from build123d import *

# Parameters (mm, degrees)
SKETCH_1_W          = 40
SKETCH_1_H          = 70
EXTRUDE_1_DEPTH     = 3
SKETCH_2_R          = 1.5
CUT_EXTRUDE_1_DEPTH = 3
CHAMFER_1_SIZE      = 0.5
CUT_EXTRUDE_2_DEPTH = 3


with BuildPart() as part:
    # 草图1 → 凸台-拉伸1 (new body)
    with BuildSketch(Plane(origin=(0, 0, 0), x_dir=(1, 0, 0), z_dir=(0, 1, 0))):
        Rectangle(SKETCH_1_W, SKETCH_1_H)
    extrude(amount=EXTRUDE_1_DEPTH)

    # 草图2 → 切除-拉伸1 (cut)
    with BuildSketch(Plane(origin=(0, 3, 0), x_dir=(1, 0, 0), z_dir=(0, 1, 0))):
        with Locations(Location((-17, 32, 0), (0, 0, 270))):
            Circle(SKETCH_2_R)
        with Locations(Location((-17, -32, 0), (0, 0, 270))):
            Circle(SKETCH_2_R)
        with Locations(Location((17, 32, 0), (0, 0, 270))):
            Circle(SKETCH_2_R)
        with Locations(Location((17, -32, 0), (0, 0, 270))):
            Circle(SKETCH_2_R)
    extrude(amount=-CUT_EXTRUDE_1_DEPTH, mode=Mode.SUBTRACT)

    # 倒角1
    chamfer_1_edges = [part.edges().sort_by_distance(p)[0] for p in [
        (-17, 0, 30.5),
        (17, 0, -33.5),
        (17, 0, 30.5),
        (-17, 0, -33.5),
    ]]
    chamfer(chamfer_1_edges, length=CHAMFER_1_SIZE)

    # 草图3 → 切除-拉伸2 (cut)
    with BuildSketch(Plane(origin=(0, 3, 0), x_dir=(1, 0, 0), z_dir=(0, 1, 0))):
        Polygon((-17, 28), (-17, 5), (-3, 28), align=None)
        Polygon((-2.622834476, 20.926536493), (-6.262463104, 14.947146604), (-2.622834476, 12.731720482), align=None)
        Polygon((-8.320477478, 12.687787001), (-2.483236099, 9.134683552), (-5, 5), (-13, 5), align=None)
        Polygon((-2.032840116, 6.708397111), (-3.07273401, 5), (-2.032840116, 5), align=None)
        Polygon((3.07273401, 5), (2.032840116, 5), (2.032840116, 6.708397111), align=None)
        Polygon((5, 5), (13, 5), (8.320477478, 12.687787001), (2.483236099, 9.134683552), align=None)
        Polygon((6.262463104, 14.947146604), (2.622834476, 12.731720482), (2.622834476, 20.926536493), align=None)
        Polygon((17, 5), (3, 28), (17, 28), align=None)
        Polygon((2.032840116, -6.708397111), (3.07273401, -5), (2.032840116, -5), align=None)
        Polygon((-3.07273401, -5), (-2.032840116, -5), (-2.032840116, -6.708397111), align=None)
        Polygon((2.483236099, -9.134683552), (5, -5), (13, -5), (8.320477478, -12.687787001), align=None)
        Polygon((-5, -5), (-13, -5), (-8.320477478, -12.687787001), (-2.483236099, -9.134683552), align=None)
        Polygon((-6.262463104, -14.947146604), (-2.622834476, -12.731720482), (-2.622834476, -20.926536493), align=None)
        Polygon((2.622834476, -20.926536493), (6.262463104, -14.947146604), (2.622834476, -12.731720482), align=None)
        Polygon((17, -28), (17, -5), (3, -28), align=None)
        Polygon((-17, -5), (-3, -28), (-17, -28), align=None)
    extrude(amount=-CUT_EXTRUDE_2_DEPTH, mode=Mode.SUBTRACT)


solid = part.part
Can you work these out from the model? Positions are in its coordinate system, mm. A direction names the side the tool comes from. Coordinates: 2 decimals unless noted, no trailing zeros. Loops run counter-clockwise (first coordinate to the right, second up) from the corner with the lowest first, then second, coordinate; pieces in that order, holes last. Notation, with made-up numbers: M 81.5,-39 L 127.5,-39 A25 ccw 127.5,-10 Z; hole C 31.25,34 d7. An arc over 180 degrees is marked long. Return JSON: item names as keys, results as strings. Group by question number.
Item 1: Thinking about a two-plate mould opening in Z: for faces 3 (the flat face through (9, 2, -5)), 4 (the flat face through (-20, 1, 0)), which applies, released by +Z, released by -Z, zero draft, split by the parting line, or undercut?
Item 2: Imagine slicing it at C-C (y = 2.3). Give the number of separate pieces and of enclosed holes in the cut face, and give its area (3 significant figures).
Item 3: Imagine slicing it at A-A (z = -32). Please give me the cut outline in (x, y).
Item 4: Imagine slicing it at B-B (x = 11.5). Please give me the cut outline in (y, z), and give its area (3 significant figures).
Item 5: If I drill on L1, parallel to X at y = 2.45, z = 32; L2, parallel to Z at x = -12, y = 1.1; L3, parallel to X at y = 0.5, z = 19, over which ranges is the centre line in solid material (lowest first)? Write a range as from..to.
Item 6: On a 3-axis mill with a long thin cutter (end or side, diameter ignored), from which of +Z, -Z, +X, -X, +Y, -Y can I reach the whole of each face in a straight line? I mean faces 1 (the flat face through (2.623, 2, 17)), 2 (the flat face through (0, 0, 0)). Say none if no direction works.
Verdict:
{
 "1": {"face 3": "undercut", "face 4": "zero draft"},
 "2": {"separate pieces": "1", "enclosed holes": "20", "area": "1,880 mm^2"},
 "3": {"outline": "M -20,0 L -19,0 L -18.5,0.5 L -18.5,3 L -20,3 Z; M -15.5,0.5 L -15,0 L 15,0 L 15.5,0.5 L 15.5,3 L -15.5,3 Z; M 18.5,0.5 L 19,0 L 20,0 L 20,3 L 18.5,3 Z"},
 "4": {"outline": "M 0,-35 L 3,-35 L 3,-28 L 0,-28 Z; M 0,-14.04 L 3,-14.04 L 3,-7.46 L 0,-7.46 Z; M 0,-5 L 3,-5 L 3,5 L 0,5 Z; M 0,7.46 L 3,7.46 L 3,14.04 L 0,14.04 Z; M 0,28 L 3,28 L 3,35 L 0,35 Z", "area": "111 mm^2"},
 "5": {"L1": "x = -20..-18.5, -15.5..15.5, 18.5..20", "L2": "z = -35..-28, -13.21..-6.64, -5..5, 6.64..13.21, 28..35", "L3": "x = -20..-17, -8.48..-3.8, -2.62..2.62, 3.8..8.48, 17..20"},
 "6": {"face 1": "+Y, -Y", "face 2": "+Z, -Z, +X, -X, -Y"}
}
